from build123d import *

# Parameters (mm, degrees)
F0_W     = 25.4
F0_H     = 31.75
F1_DEPTH = 31.75
F2_R     = 7.9375
F3_DEPTH = 31.75
F5_DEPTH = 31.75


with BuildPart() as f1:
    # F0 (on Front) → F1 (new body)
    with BuildSketch(Plane.XZ):
        Rectangle(F0_W, F0_H)
    extrude(amount=F1_DEPTH)

    # F2 (on face) → F3 (cut, through all)
    with BuildSketch(Plane(origin=(0, 0, 0), x_dir=(-1, 0, 0), z_dir=(0, 1, 0))):
        with Locations((0, -3.175)):
            Circle(F2_R)
    extrude(amount=-F3_DEPTH, mode=Mode.SUBTRACT)

    # F4 (on face) → F5 (join, through all)
    with BuildSketch(Plane(origin=(0, 0, 0), x_dir=(-1, 0, 0), z_dir=(0, 1, 0))):
        Polygon((19.05, 15.875), (-19.05, 15.875), (-12.707431, 9.532431), (12.707431, 9.532431), align=None)
    extrude(amount=-F5_DEPTH)


solid = f1.part
For this review, take the finished solid that the model builds, in its own axes (mm). A direction names the side the tool comes from. Give positions to 0.01 mm unless a question says otherwise; leave off trailing zeros. Order: outer loops, then holes, each group sorted by start corner. A loop starts at its lowest first (then second) coordinate and runs counter-clockwise, first axis right, second up. Notation, with made-up numbers: (7.5, 45.25) -> (17.5, 45.25) arc R11 ccw to (17.5, 60.25) -> close; hole circle Ø2 at (88, -14.5). An arc over 180 degrees is marked (long way). Write item = value, one per line.
1) Draft analysis for pull direction X (two halves, no side actions). For faces 1 (the face through (0, -16, -15.875)), 2 (the face through (1.721, -15.653, -10.924)), 3 (the face through (12.7, -16, -3)), state which applies: pulls with the +X half, pulls with the -X half, needs draft (parallel to the pull), parting line crosses it, or undercut.
Findings:
face_1 = needs draft
face_2 = undercut
face_3 = pulls with the +X half
2) We need section B-B, the plane z = -10. Give the boundary of the cut face in (x, y), and give its area (3 significant figures).
Findings:
outline = (-12.7, -31.75) -> (-4.05, -31.75) -> (-4.05, 0) -> (-12.7, 0) -> close; (4.05, -31.75) -> (12.7, -31.75) -> (12.7, 0) -> (4.05, 0) -> close
area = 549 mm^2
3) For faces 4 (the face through (-12.7, -16, -3)), 5 (the face through (15.923, -15.653, 12.748)), list the 3-axis set-ups (+Z, -Z, +X, -X, +Y, -Y) from which the entire face can be reached by the end or side of a thin tool; tool diameter is ignored.
Findings:
face_4 = -Z, -X, +Y, -Y
face_5 = -Z, +X, +Y, -Y
4) To check wall thickness, follow L1, parallel to Z at x = 0, y = -17.5 (1 decimal); L2, parallel to X at y = -24, z = 8; L3, parallel to X at y = -14, z = -1. State the ranges of each line that lie inside material, in increasing order. Write a range as from..to.
Findings:
L1 = -15.9..-11.1, 4.8..15.9
L2 = -12.7..12.7
L3 = -12.7..-7.63, 7.63..12.7
5) Insertion check: pin 1 (5 mm diameter, centred on x = 6, z = 8, fed in from +Y); pin 2 (7.5 mm diameter, centred on y = -8.5, z = -4, fed in from +X); pin 3 (8 mm diameter, centred on y = -16, z = 5, fed in from -X); pin 4 (10 mm diameter, centred on y = -18, z = 5, fed in from +X) (3 decimals). Each pin has a flat end and moves straight along its axis. Give the tip position at first contact, or say it passes through.
Findings:
pin_1 = 0
pin_2 = 12.7
pin_3 = -12.7
pin_4 = 13.175
